Input: part model. Units: mm. Frame: model coordinates. A direction names the side the tool comes from. Coordinates: 2 decimals unless noted, no trailing zeros. Loops run counter-clockwise (first coordinate to the right, second up) from the corner with the lowest first, then second, coordinate; pieces in that order, holes last. Notation, with made-up numbers: (75, 1.25) -> (112, 1.25) arc R8 cw to (112, 15.25) -> close; hole circle Ø9 at (81.5, 6). An arc over 180 degrees is marked (long way). Put each result on its own line as item: value. Start each with the question number.
1) Pull-direction query (Y, two-part tool) for faces 1 (the flat face through (1, 34.623, -22)), 2 (the flat face through (1, 53, 3.615)), 3 (the flat face through (1, 12.623, 16)); classes: pulls with the +Y half, pulls with the -Y half, needs draft (parallel to the pull), parting line crosses it, or undercut.
2) Material intervals for L1, parallel to Y at x = 0.35, z = -13.5; L2, parallel to Y at x = 2.25, z = 9.5; L3, parallel to Z at x = 0.65, y = 6.5, sorted ascending.
3) Contact query for flat-ended pins moving along their axis: P1, Ø1.5, axis at x = 1, y = 17, coming from the -Z side; P2, Ø1, axis at x = 1, z = 16, coming from the +Y side; P3, Ø1.1, axis at x = 2, y = -14, coming from the +Z side; P4, Ø8, axis at y = -32.5, z = 17.5, coming from the -X side. Output: stop coordinate, or through.
4) Set-up query: faces 4 (the flat face through (1, -54, 13.615)), 5 (the flat face through (1, 53, -3.385)), 6 (the flat face through (1, -17.377, 16)), 7 (the flat face through (1, -16.377, 19)), 8 (the flat face through (1, 13.623, -19)). Return all of +Z, -Z, +X, -X, +Y, -Y with unobstructed straight access to the full face (end or side cutting, diameter ignored); none if empty.
5) Cut plane A-A (y = 47.5). Return the cut outline in (x, z), plus the area to 3 significant figures.
from build123d import *

# Parameters (mm, degrees)
F1_DEPTH = 3


with BuildPart() as f1:
    # F0 (on Right) → F1 (new body)
    with BuildSketch(Plane.YZ):
        Polygon((-52.377451, -13.384804), (-52.377451, -20.384804), (-35.377451, -20.384804), (-35.377451, -23.384804), (-25.377451, -23.384804), (-25.377451, -20.384804), (-16.377451, -20.384804), (-16.377451, -16.884804), (-17.377451, -16.884804), (-17.377451, -14.884804), (-16.377451, -14.884804), (-16.377451, -8.384804), (-14.377451, -8.384804), (-14.377451, -14.884804), (-13.377451, -14.884804), (-13.377451, -16.884804), (-14.377451, -16.884804), (-14.377451, -20.384804), (-5.377451, -20.384804), (-5.377451, -23.384804), (-0.377451, -23.384804), (4.622549, -23.384804), (4.622549, -20.384804), (13.622549, -20.384804), (13.622549, -16.884804), (12.622549, -16.884804), (12.622549, -14.884804), (13.622549, -14.884804), (13.622549, -8.384804), (15.622549, -8.384804), (15.622549, -14.884804), (16.622549, -14.884804), (16.622549, -16.884804), (15.622549, -16.884804), (15.622549, -20.384804), (24.622549, -20.384804), (24.622549, -23.384804), (34.622549, -23.384804), (34.622549, -20.384804), (51.622549, -20.384804), (51.622549, -13.384804), (54.622549, -13.384804), (54.622549, -3.384804), (51.622549, -3.384804), (51.622549, 0.115196), (51.622549, 3.615196), (54.622549, 3.615196), (54.622549, 13.615196), (51.622549, 13.615196), (51.622549, 20.615196), (34.622549, 20.615196), (34.622549, 23.615196), (24.622549, 23.615196), (24.622549, 20.615196), (15.622549, 20.615196), (15.622549, 17.115196), (16.622549, 17.115196), (16.622549, 15.115196), (15.622549, 15.115196), (15.622549, 8.615196), (13.622549, 8.615196), (13.622549, 15.115196), (12.622549, 15.115196), (12.622549, 17.115196), (13.622549, 17.115196), (13.622549, 20.615196), (4.622549, 20.615196), (4.622549, 23.615196), (-0.377451, 23.615196), (-5.377451, 23.615196), (-5.377451, 20.615196), (-14.377451, 20.615196), (-14.377451, 17.115196), (-13.377451, 17.115196), (-13.377451, 15.115196), (-14.377451, 15.115196), (-14.377451, 8.615196), (-16.377451, 8.615196), (-16.377451, 15.115196), (-17.377451, 15.115196), (-17.377451, 17.115196), (-16.377451, 17.115196), (-16.377451, 20.615196), (-25.377451, 20.615196), (-25.377451, 23.615196), (-35.377451, 23.615196), (-35.377451, 20.615196), (-52.377451, 20.615196), (-52.377451, 13.615196), (-55.377451, 13.615196), (-55.377451, 3.615196), (-52.377451, 3.615196), (-52.377451, 0.115196), (-52.377451, -3.384804), (-55.377451, -3.384804), (-55.377451, -13.384804), align=None)
    extrude(amount=F1_DEPTH)


solid = f1.part
Results found:
1. face 1: pulls with the +Y half
1. face 2: needs draft
1. face 3: undercut
2. L1: y = -52.38 to -16.38, -14.38 to 13.62, 15.62 to 51.62
2. L2: y = -55.38 to -16.38, -14.38 to 13.62, 15.62 to 54.62
2. L3: z = -20.38 to 20.62
3. P1: stops at z = -20.38
3. P2: stops at y = 51.62
3. P3: stops at z = 20.62
3. P4: stops at x = 0
4. face 4: +Z, +X, -X, -Y
4. face 5: +X, -X, +Y
4. face 6: +X, -X
4. face 7: +Z, +X, -X
4. face 8: -Z, +X, -X
5. outline: (0, -20.38) -> (3, -20.38) -> (3, 20.62) -> (0, 20.62) -> close
5. area: 123 mm2
